```python
from build123d import *

# Parameters (mm, degrees)
SKETCH1_R                   = 8.7
BOSS_EXTRUDE1_DEPTH         = 29.5
SKETCH5_R                   = 1.75
CUT_EXTRUDE1_DEPTH          = 32.962947298
SKETCH6_R                   = 3.05
CUT_EXTRUDE3_DEPTH          = 26.5
SKETCH2_W                   = 17
SKETCH2_H                   = 4.566888769
CUT_EXTRUDE4_DEPTH          = 11
FILLET1_R                   = 0.3
TAP_DRILL_FOR_M3X0_5_TAP1_D = 2.5
SKETCH4_R                   = 2
BOSS_EXTRUDE2_DEPTH         = 3


with BuildPart() as part:
    # Sketch1 → Boss-Extrude1 (new body)
    with BuildSketch(Plane.XY):
        Circle(SKETCH1_R)
    extrude(amount=BOSS_EXTRUDE1_DEPTH)

    # Sketch5 → Cut-Extrude1 (cut, through all)
    with BuildSketch(Plane(origin=(0, 0, 0), x_dir=(-1, 0, 0), z_dir=(0, 0, -1))):
        Circle(SKETCH5_R)
    extrude(amount=-CUT_EXTRUDE1_DEPTH, mode=Mode.SUBTRACT)

    # Sketch6 → Cut-Extrude3 (cut)
    with BuildSketch(Plane.XY.offset(29.5)):
        Circle(SKETCH6_R)
    extrude(amount=-CUT_EXTRUDE3_DEPTH, mode=Mode.SUBTRACT)

    # Sketch2 → Cut-Extrude4 (cut)
    with BuildSketch(Plane.XY.offset(29.5)):
        with Locations((0.844453543, 6.416555616)):
            Rectangle(SKETCH2_W, SKETCH2_H)
    extrude(amount=-CUT_EXTRUDE4_DEPTH, mode=Mode.SUBTRACT)

    # Fillet1
    fillet1_edges = [part.edges().sort_by_distance(p)[0] for p in [
        (1.75, 0, 3),
    ]]
    fillet(fillet1_edges, radius=FILLET1_R)

    # Tap Drill for M3x0.5 Tap1 (through all)
    with Locations(Plane(origin=(0, 4.133111231, 0), x_dir=(1, 0, 0), z_dir=(0, 1, 0))):
        with Locations((4.644453543, -24), (-4.355546457, -24)):
            Hole(TAP_DRILL_FOR_M3X0_5_TAP1_D / 2)

    # Sketch4 → Boss-Extrude2 (add)
    with BuildSketch(Plane(origin=(0, 0, 0), x_dir=(-1, 0, 0), z_dir=(0, 0, -1))):
        with Locations(Location((0, 6, 0), (0, 0, 180))):
            Circle(SKETCH4_R)
        with Locations(Location((6, 0, 0), (0, 0, 180))):
            Circle(SKETCH4_R)
        with Locations(Location((0, -6, 0), (0, 0, 180))):
            Circle(SKETCH4_R)
        with Locations(Location((-6, 0, 0), (0, 0, 180))):
            Circle(SKETCH4_R)
    extrude(amount=BOSS_EXTRUDE2_DEPTH)


solid = part.part
```
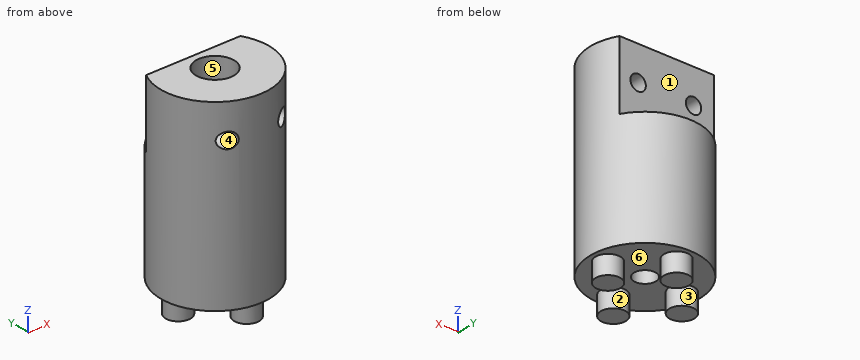
Geometry check sheet. Reference: the model listing, model coordinates, mm. Face numbers are marked on the shaded views. A direction names the side the tool comes from. Give positions to 0.01 mm unless a question says otherwise; leave off trailing zeros. Order: outer loops, then holes, each group sorted by start corner. A loop starts at its lowest first (then second) coordinate and runs counter-clockwise, first axis right, second up.
1. Section check C-C, the plane z = 24. Enter the section's corners in (x, y).
2. Access from +Z, -Z, +X, -X, +Y, -Y to the whole of each face (thin tool, end or side, straight path). Record for the marked faces 4, 5 and 6.
3. Release check for a two-part mould opening along X. For the marked faces 1, 2 and 3 record: pulls with the +X half, pulls with the -X half, needs draft (parallel to the pull), parting line crosses it, or undercut.
4. Gauge pin test, flat ends, axial feed: pin 1 Ø1.5 at (x, z) = (2.5, 18.5) entering from -Y; pin 2 Ø3 at (x, z) = (-3, 20.5) entering from +Y; pin 3 Ø1 at (y, z) = (-2.5, 1.5) entering from +X; pin 4 Ø1.5 at (x, z) = (4.64, 24) entering from -Y. Record the tip position at first contact, or that the pin passes through.
5. Section check D-D, the plane y = 6. Enter the section's corners in (x, z), and give its area (3 significant figures).
6. Thickness scan on L1, parallel to Y at x = 0, z = 11.5; L2, parallel to Z at x = -4.5, y = 4; L3, parallel to Z at x = -6.25, y = 4.5. Record the ranges inside material, lowest first.
7. Section check A-A, the plane y = 0. Enter the section's corners in (x, z).
8. Section check B-B, the plane x = 0. Enter the section's corners in (y, z).
Values follow:
1. outline: (-7.66, 4.13) arc R8.7 ccw to (-5.61, -6.65) - (-5.61, 4.13) - close; (-3.11, -8.13) arc R8.7 ccw to (3.39, -8.01) - (3.39, 4.13) - (-3.11, 4.13) - close; (5.89, -6.4) arc R8.7 ccw to (7.66, 4.13) - (5.89, 4.13) - close; hole circle Ø6.1 at (0, 0)
2. face 4: +Y, -Y
2. face 5: +Z
2. face 6: -Z
3. face 1: needs draft
3. face 2: parting line crosses it
3. face 3: undercut
4. pin 1: stops at y = -8.52
4. pin 2: stops at y = 4.13
4. pin 3: stops at x = 8.47
4. pin 4: passes through
5. outline: (-6.3, 0) - (-2, 0) - (-2, -3) - (2, -3) - (2, 0) - (6.3, 0) - (6.3, 18.5) - (-6.3, 18.5) - close
5. area: 245 mm2
6. L1: y = -8.7 to -3.05, 3.05 to 8.7
6. L2: z = 0 to 22.76, 25.24 to 29.5
6. L3: z = 0 to 18.5
7. outline: (-8.7, 0) - (-8, 0) - (-8, -3) - (-4, -3) - (-4, 0) - (-1.75, 0) - (-1.75, 2.7) arc R0.3 ccw to (-2.05, 3) - (-3.05, 3) - (-3.05, 29.5) - (-8.7, 29.5) - close; (1.75, 0) - (4, 0) - (4, -3) - (8, -3) - (8, 0) - (8.7, 0) - (8.7, 29.5) - (3.05, 29.5) - (3.05, 3) - (2.05, 3) arc R0.3 ccw to (1.75, 2.7) - close; hole circle Ø2.5 at (-4.36, 24); hole circle Ø2.5 at (4.64, 24)
8. outline: (-8.7, 0) - (-8, 0) - (-8, -3) - (-4, -3) - (-4, 0) - (-1.75, 0) - (-1.75, 2.7) arc R0.3 ccw to (-2.05, 3) - (-3.05, 3) - (-3.05, 29.5) - (-8.7, 29.5) - close; (1.75, 0) - (4, 0) - (4, -3) - (8, -3) - (8, 0) - (8.7, 0) - (8.7, 18.5) - (4.13, 18.5) - (4.13, 29.5) - (3.05, 29.5) - (3.05, 3) - (2.05, 3) arc R0.3 ccw to (1.75, 2.7) - close
